Read the model definition and answer for the solid it produces. Units are mm, in the model's axes. Face numbers are marked on the shaded views. Give positions to 0.01 mm unless a question says otherwise; leave off trailing zeros. Order: outer loops, then holes, each group sorted by start corner. A loop starts at its lowest first (then second) coordinate and runs counter-clockwise, first axis right, second up. Notation, with made-up numbers: (-24.5, 10) -> (-0.5, 10) arc R31 ccw to (-0.5, 39) -> close; hole circle Ø1 at (58, -7). An arc over 180 degrees is marked (long way). One line per question, with ' | ' between items. Start each with the question number.
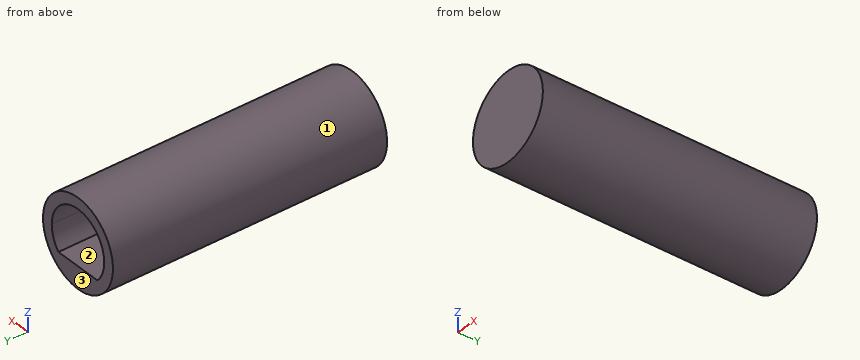
```python
from build123d import *

# Parameters (mm, degrees)
F0_R     = 4
F1_DEPTH = 25
F2_DEPTH = 10


with BuildPart() as f1:
    # F0 (on Front) → F1 (new body)
    with BuildSketch(Plane.XZ):
        Circle(F0_R)
        with BuildLine():
            ThreePointArc((-2.2360679775, -2), (-1.0704662693, 2.8025170769), (3, 0))
            ThreePointArc((3, 0), (2.8025170769, -1.0704662693), (2.2360679775, -2))
            ThreePointArc((2.2360679775, -2), (1.2247448714, -2.7386127875), (0, -3))
            ThreePointArc((0, -3), (-1.2247448714, -2.7386127875), (-2.2360679775, -2))
        make_face(mode=Mode.SUBTRACT)
        with BuildLine():
            ThreePointArc((2.2360679775, -2), (2.8025170769, -1.0704662693), (3, 0))
            ThreePointArc((3, 0), (-1.0704662693, 2.8025170769), (-2.2360679775, -2))
            Line((-2.2360679775, -2), (0, -2))
            Line((0, -2), (2.2360679775, -2))
        make_face()
        with BuildLine():
            ThreePointArc((0, -3), (1.2247448714, -2.7386127875), (2.2360679775, -2))
            Line((2.2360679775, -2), (0, -2))
            Line((0, -2), (0, -3))
        make_face()
        with BuildLine():
            Line((0, -2), (-2.2360679775, -2))
            ThreePointArc((-2.2360679775, -2), (-1.2247448714, -2.7386127875), (0, -3))
            Line((0, -3), (0, -2))
        make_face()
    extrude(amount=F1_DEPTH)

    # F0 (on Front) → F2 (cut)
    with BuildSketch(Plane.XZ):
        with BuildLine():
            ThreePointArc((2.2360679775, -2), (2.8025170769, -1.0704662693), (3, 0))
            ThreePointArc((3, 0), (-1.0704662693, 2.8025170769), (-2.2360679775, -2))
            Line((-2.2360679775, -2), (0, -2))
            Line((0, -2), (2.2360679775, -2))
        make_face()
    extrude(amount=F2_DEPTH, mode=Mode.SUBTRACT)


solid = f1.part
```
Q1. A cutting plane is placed at A-A, the plane x = 0. Determine the outline of the cut face in (y, z), then the cut area to 3 significant figures.
Q2. Find the intervals of material crossed by line 1 (Z direction, x = 0, y = -6.75); line 2 (Y direction, x = 0.5, z = -1); line 3 (Z direction, x = 1.5, y = -4.5), in increasing order.
Q3. Given P1, Ø1, axis at y = -19, z = 1, coming from the -X side; P2, Ø3, axis at x = -2, y = -16, coming from the +Z side, each flat-ended and moving along its own axis, determine where each tip first touches the part or whether it passes through.
Q4. Determine the mould class of the marked faces 1, 2 and 3 for opening direction X: pulls with the +X half, pulls with the -X half, needs draft (parallel to the pull), parting line crosses it, or undercut.
Q5. A cutting plane is placed at C-C, the plane y = -7. Determine the outline of the cut face in (x, z), then the cut area to 3 significant figures.
Q6. A cutting plane is placed at D-D, the plane y = -13.75. Determine the outline of the cut face in (x, z), then the cut area to 3 significant figures.
Q7. A cutting plane is placed at B-B, the plane z = 1.5. Determine the outline of the cut face in (x, y), then the cut area to 3 significant figures.
Geometry results:
1) outline: (-25, -4) -> (0, -4) -> (0, -2) -> (-10, -2) -> (-10, 3) -> (0, 3) -> (0, 4) -> (-25, 4) -> close | area: 150 mm²
2) line 1: -4 to -2, 3 to 4 | line 2: -25 to -10 | line 3: -3.71 to -2, 2.6 to 3.71
3) P1: x = -3.97 | P2: z = 3.97
4) face 1: parting line crosses it | face 2: undercut | face 3: needs draft
5) outline: circle Ø8 at (0, 0); hole (-2.24, -2) -> (2.24, -2) arc R3 ccw (long way) to start | area: 25.1 mm²
6) outline: circle Ø8 at (0, 0) | area: 50.3 mm²
7) outline: (-3.71, -25) -> (3.71, -25) -> (3.71, 0) -> (2.6, 0) -> (2.6, -10) -> (-2.6, -10) -> (-2.6, 0) -> (-3.71, 0) -> close | area: 133 mm²
